Can you work these out from the model? Positions are in its coordinate system, mm. Face numbers are marked on the shaded views. A direction names the side the tool comes from. Give positions to 0.01 mm unless a question says otherwise; leave off trailing zeros. Loops run counter-clockwise (first coordinate to the right, second up) from the corner with the lowest first, then second, coordinate; pieces in that order, holes last. Notation, with made-up numbers: M -22,42 L 10,42 A24 ccw 10,63 Z; hole C 60,-7 d10. An arc over 180 degrees is marked long. Put each result on its own line as item: value. Start each with the question number.
1) For P1, Ø8, axis at x = -6.5, z = 23, coming from the +Y side; P2, Ø12, axis at y = 28.5, z = 4, coming from the +X side; P3, Ø6, axis at x = 9.5, y = 17.5, coming from the +Z side, each with a flat end and sliding along its axis, tell me the tip position at first contact or that it passes through.
2) Imagine slicing it at A-A (z = 11). Write out the boundary of the cut face in (x, y).
3) For the marked faces 1 and 2, which set-ups out of +Z, -Z, +X, -X, +Y, -Y let a thin tool reach every point of the face, with its end or its side?
4) Imagine slicing it at C-C (x = 0.5). Write out the boundary of the cut face in (y, z).
5) Imagine slicing it at B-B (z = 22). Write out the boundary of the cut face in (x, y), then the cut area to 3 significant figures.
6) If we mould it in two halves opening along X, with no side actions, what happens to the marked faces 3, 4 and 5? For each: +X half, -X half, draft (parallel to the pull), parting line (faces both ways), or undercut.
7) Imagine slicing it at D-D (x = 8). Write out the boundary of the cut face in (y, z).
8) Please list where these lines run through material, in increasing order: line 1 along X through (y, z) = (1.1, 11); line 2 along Z through (x, y) = (-3, 25). Write a range as from..to.
from build123d import *

# Parameters (mm, degrees)
SKETCH_1_W      = 26.5
SKETCH_1_H      = 33
SKETCH_1_R      = 5
SKETCH_1_R_2    = 1.5
EXTRUDE_1_DEPTH = 3
SKETCH_2_R      = 4
SKETCH_2_R_2    = 1.5
EXTRUDE_2_DEPTH = 3


with BuildPart() as part:
    # 草图1 → 凸台-拉伸1 (new body)
    with BuildSketch(Plane(origin=(0, 0, 0), x_dir=(1, 0, 0), z_dir=(0, 1, 0))):
        with Locations((0, -16.5)):
            Rectangle(SKETCH_1_W, SKETCH_1_H)
        with Locations(Location((0, -18, 0), (0, 0, 270))):
            Circle(SKETCH_1_R, mode=Mode.SUBTRACT)
        with Locations(Location((-8, -11, 0), (0, 0, 270))):
            Circle(SKETCH_1_R_2, mode=Mode.SUBTRACT)
        with Locations(Location((8, -11, 0), (0, 0, 270))):
            Circle(SKETCH_1_R_2, mode=Mode.SUBTRACT)
        with Locations(Location((-8, -25, 0), (0, 0, 270))):
            Circle(SKETCH_1_R_2, mode=Mode.SUBTRACT)
        with Locations(Location((8, -25, 0), (0, 0, 270))):
            Circle(SKETCH_1_R_2, mode=Mode.SUBTRACT)
    extrude(amount=EXTRUDE_1_DEPTH)

    # 草图2 → 凸台-拉伸2 (add)
    with BuildSketch(Plane.XY):
        with BuildLine():
            Line((-13.25, 3), (-13.25, 19.75))
            ThreePointArc((-13.25, 19.75), (0, 33), (13.25, 19.75))
            Line((13.25, 19.75), (13.25, 3))
            Line((13.25, 3), (-13.25, 3))
        make_face()
        with Locations((0, 19.75)):
            Circle(SKETCH_2_R, mode=Mode.SUBTRACT)
        with Locations((-8.5, 19.75)):
            Circle(SKETCH_2_R_2, mode=Mode.SUBTRACT)
        with Locations((8.5, 19.75)):
            Circle(SKETCH_2_R_2, mode=Mode.SUBTRACT)
    extrude(amount=EXTRUDE_2_DEPTH)


solid = part.part
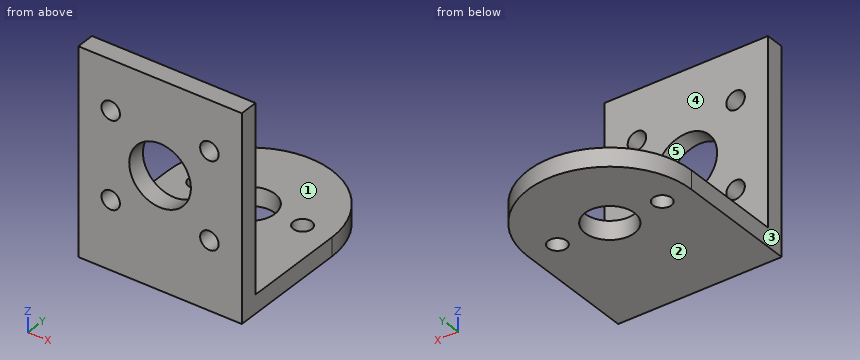
Recorded:
1. P1: y = 3
1. P2: x = 12.94
1. P3: z = 3
2. outline: M -13.25,0 L -9.5,0 L -9.5,3 L -13.25,3 Z; M -6.5,0 L 6.5,0 L 6.5,3 L -6.5,3 Z; M 9.5,0 L 13.25,0 L 13.25,3 L 9.5,3 Z
3. face 1: +Z, +X, -X, +Y
3. face 2: -Z, +X, -X, +Y, -Y
4. outline: M 0,0 L 15.78,0 L 15.78,3 L 3,3 L 3,13.03 L 0,13.03 Z; M 0,22.97 L 3,22.97 L 3,33 L 0,33 Z; M 23.72,0 L 32.99,0 L 32.99,3 L 23.72,3 Z
5. outline: M -13.25,0 L -3,0 L -3,3 L -13.25,3 Z; M 3,0 L 13.25,0 L 13.25,3 L 3,3 Z
5. area: 61.5 mm²
6. face 3: -X half
6. face 4: draft
6. face 5: undercut
7. outline: M 0,0 L 18.34,0 L 18.34,3 L 3,3 L 3,9.5 L 0,9.5 Z; M 0,12.5 L 3,12.5 L 3,23.5 L 0,23.5 Z; M 0,26.5 L 3,26.5 L 3,33 L 0,33 Z; M 21.16,0 L 30.31,0 L 30.31,3 L 21.16,3 Z
8. line 1: -13.25..-9.5, -6.5..6.5, 9.5..13.25
8. line 2: 0..3
